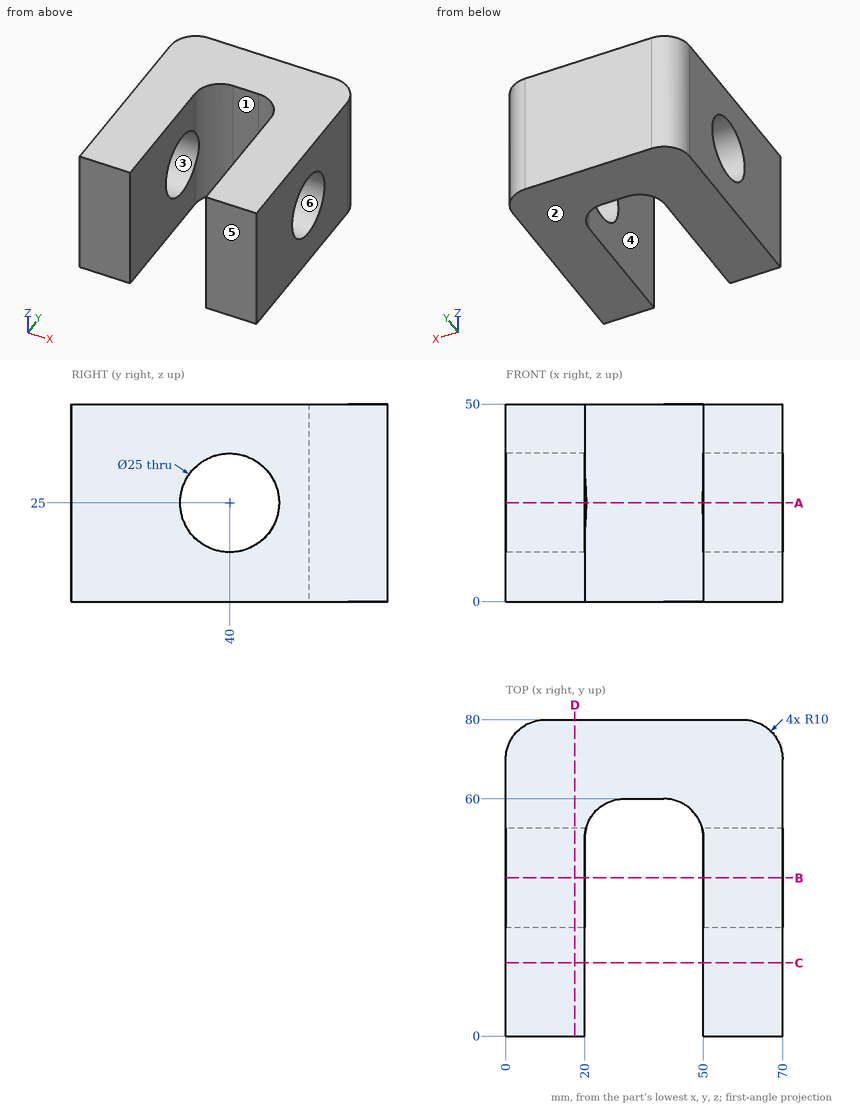
Can you work these out from the drawing? Everything is in mm from the part's minimum corner. A direction names the side the tool comes from. Round coordinates to 2 decimals unless told otherwise and drop trailing zeros. Loops run counter-clockwise (first coordinate to the right, second up) from the corner with the lowest first, then second, coordinate; pieces in that order, holes last. Notation, with made-up numbers: (37, 44.5) -> (81, 44.5) arc R27 ccw to (81, 61.5) -> close; hole circle Ø5 at (44.5, 14). An arc over 180 degrees is marked (long way). Use CSV: the item, a comma, the result in double quotes.
(1) Suppose I cut it at D-D on x = 17.5. Write out the boundary of the cut face in (y, z).
Return value:
outline,"(0, 0) -> (80, 0) -> (80, 50) -> (0, 50) -> close; hole circle Ø25 at (40, 25)"
(2) If we mould it in two halves opening along Y, with no side actions, what happens to the marked faces 3, 4, 5 and 6? For each: +Y half, -Y half, draft (parallel to the pull), parting line (faces both ways), or undercut.
Return value:
face 3,"undercut"
face 4,"draft"
face 5,"-Y half"
face 6,"undercut"
(3) Suppose I cut it at C-C on y = 18.5. Write out the boundary of the cut face in (x, z).
Return value:
outline,"(0, 0) -> (20, 0) -> (20, 50) -> (0, 50) -> close; (50, 0) -> (70, 0) -> (70, 50) -> (50, 50) -> close"
(4) Suppose I cut it at B-B on y = 40. Write out the boundary of the cut face in (x, z).
Return value:
outline,"(0, 0) -> (20, 0) -> (20, 12.5) -> (0, 12.5) -> close; (0, 37.5) -> (20, 37.5) -> (20, 50) -> (0, 50) -> close; (50, 0) -> (70, 0) -> (70, 12.5) -> (50, 12.5) -> close; (50, 37.5) -> (70, 37.5) -> (70, 50) -> (50, 50) -> close"
(5) For the marked faces 1 and 2, which set-ups out of +Z, -Z, +X, -X, +Y, -Y let a thin tool reach every point of the face, with its end or its side?
Return value:
face 1,"+Z, -Z, -Y"
face 2,"-Z, +X, -X, +Y, -Y"
(6) Will these pins go through, and if not, where does the flat tip stop? pin 1 Ø15 at (y, z) = (40, 25) entering from -X; pin 2 Ø1.5 at (x, z) = (62, 19) entering from +Y; pin 3 Ø3 at (x, z) = (35, 16) entering from -Y.
Return value:
pin 1,"passes through"
pin 2,"stops at y = 79.92"
pin 3,"stops at y = 60"
(7) If I drill on probe 1 along X at (y, z) = (21.5, 33.5); probe 2 along Z at (x, y) = (14.25, 40); probe 3 along Z at (x, y) = (54, 42.5), over which ranges is the centre line in solid material (lowest first)? Write a range as [from, to].
Return value:
probe 1,"x = [0, 20], [50, 70]"
probe 2,"z = [0, 12.5], [37.5, 50]"
probe 3,"z = [0, 12.75], [37.25, 50]"
(8) Suppose I cut it at A-A on z = 25. Write out the boundary of the cut face in (x, y), plus the area to 3 significant figures.
Return value:
outline,"(0, 0) -> (20, 0) -> (20, 27.5) -> (0, 27.5) -> close; (0, 52.5) -> (20.32, 52.5) arc R10 cw to (30, 60) -> (40, 60) arc R10 cw to (49.68, 52.5) -> (70, 52.5) -> (70, 70) arc R10 ccw to (60, 80) -> (10, 80) arc R10 ccw to (0, 70) -> close; (50, 0) -> (70, 0) -> (70, 27.5) -> (50, 27.5) -> close"
area,"2,800 mm²"
